Could you check a few things on this drawing? It's one solid part, dimensions in mm from its lowest x, y, z. A direction names the side the tool comes from. Give positions to 0.01 mm unless a question says otherwise; leave off trailing zeros. Loops run counter-clockwise (first coordinate to the right, second up) from the corner with the lowest first, then second, coordinate; pieces in that order, holes last. Notation, with made-up numbers: (19.5, 24.25) - (51.5, 24.25) arc R20 cw to (51.5, 59.25) - close; hole circle Ø8 at (3, 44.25). An arc over 180 degrees is marked (long way). Put each result on its own line as item: value. Start each with the question number.
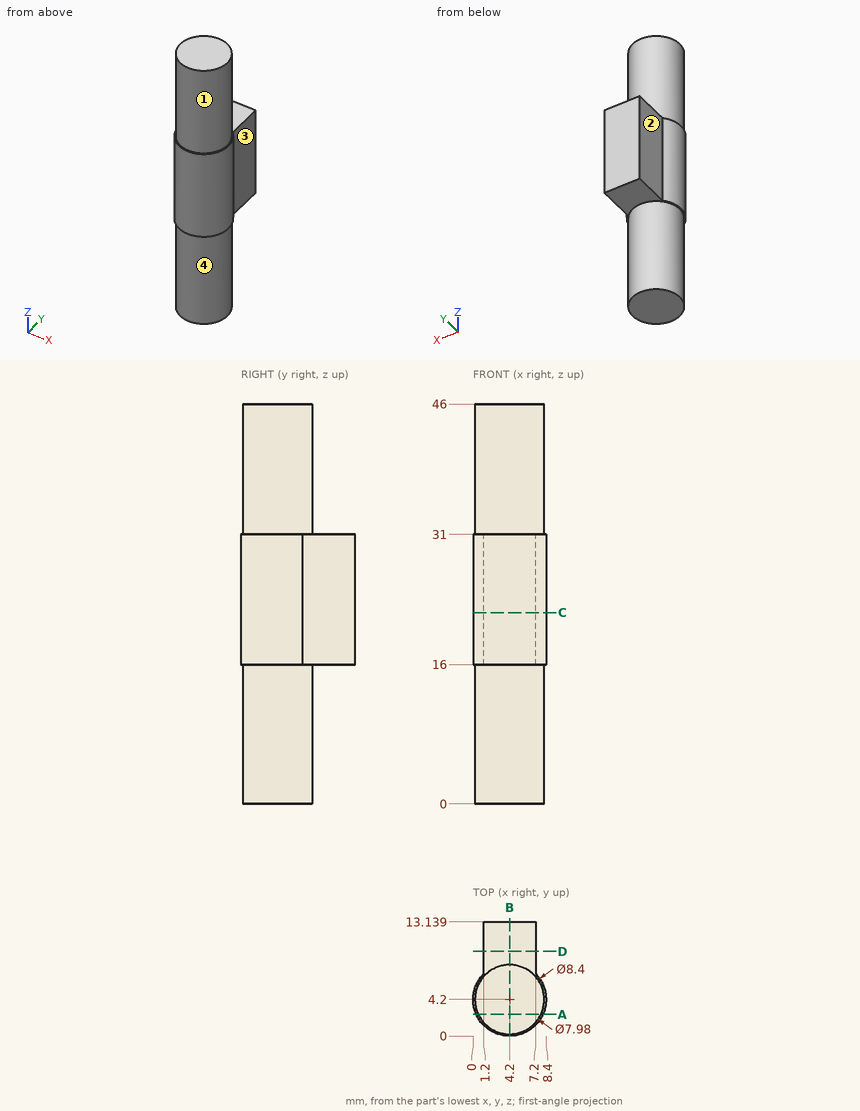
1) Suppose I cut it at C-C on z = 22. Please give me the cut outline in (x, y).
2) Suppose I cut it at D-D on y = 9.75. Please give me the cut outline in (x, z), plus the area to 3 significant figures.
3) Which directions (+Z, -Z, +X, -X, +Y, -Y) give clear straight access to the entire face, cutting with the end or side of a thin tool? Please do the marked faces 1, 2, 3 and 4.
4) I need wall thicknesses on line 1 (Z direction, x = 1.25, y = 10.75); line 2 (X direction, y = 10.75, z = 21); line 3 (X direction, y = 2, z = 43). Which ranges of each line are inside material? Lowest first, please.
5) Suppose I cut it at B-B on x = 4.2. Please give me the cut outline in (y, z).
6) I'm going to push flat-ended pins straight in: P1, Ø1.5, axis at x = 4.5, y = 11, coming from the +Z side; P2, Ø2, axis at y = 2.5, z = 39, coming from the -X side; P3, Ø3, axis at y = 10.5, z = 22.5, coming from the +X side. Where does each tip first touch, or does it pass through?
7) Suppose I cut it at A-A on y = 2.5. Please give me the cut outline in (x, z).
Ans:
1. outline: (1.2, 7.14) arc R4.2 ccw (long way) to (7.2, 7.14) - (7.2, 13.14) - (1.2, 13.14) - close
2. outline: (1.2, 16) - (7.2, 16) - (7.2, 31) - (1.2, 31) - close
2. area: 90.0 mm²
3. face 1: +Z
3. face 2: +Z, -Z, -X, +Y
3. face 3: +Z, -Z, +X, +Y
3. face 4: -Z
4. line 1: z = 16 to 31
4. line 2: x = 1.2 to 7.2
4. line 3: x = 0.87 to 7.53
5. outline: (0, 16) - (0.21, 16) - (0.21, 0) - (8.19, 0) - (8.19, 16) - (13.14, 16) - (13.14, 31) - (8.19, 31) - (8.19, 46) - (0.21, 46) - (0.21, 31) - (0, 31) - close
6. P1: stops at z = 31
6. P2: stops at x = 0.27
6. P3: stops at x = 7.2
7. outline: (0.36, 16) - (0.59, 16) - (0.59, 0) - (7.81, 0) - (7.81, 16) - (8.04, 16) - (8.04, 31) - (7.81, 31) - (7.81, 46) - (0.59, 46) - (0.59, 31) - (0.36, 31) - close
